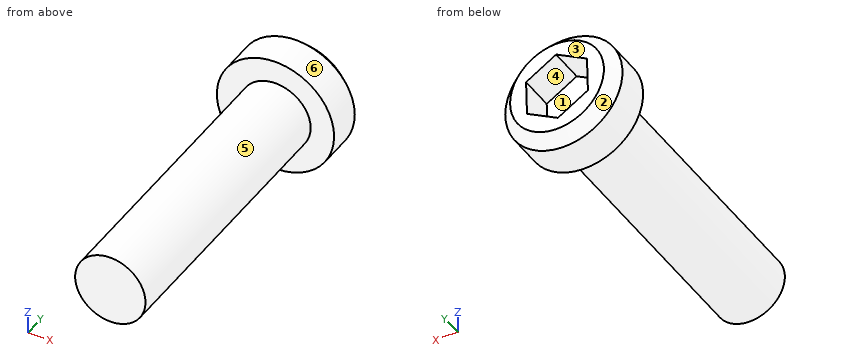
```python
from build123d import *

# Parameters (mm, degrees)
SKETCH1_R           = 1.5
BOSS_EXTRUDE1_DEPTH = 12
SKETCH2_R           = 2.5
BOSS_EXTRUDE2_DEPTH = 2
CHAMFER1_SIZE       = 0.5
CUT_EXTRUDE1_DEPTH  = 1.5


with BuildPart() as part:
    # Sketch1 → Boss-Extrude1 (new body)
    with BuildSketch(Plane(origin=(0, 0, 0), x_dir=(1, 0, 0), z_dir=(0, 1, 0))):
        with Locations((-74.537838868, 155.62707166)):
            Circle(SKETCH1_R)
    extrude(amount=-BOSS_EXTRUDE1_DEPTH)

    # Sketch2 → Boss-Extrude2 (add)
    with BuildSketch(Plane(origin=(0, 0, 0), x_dir=(1, 0, 0), z_dir=(0, 1, 0))):
        with Locations((-74.537838868, 155.62707166)):
            Circle(SKETCH2_R)
    extrude(amount=BOSS_EXTRUDE2_DEPTH)

    # Chamfer1
    chamfer1_edges = [part.edges().sort_by_distance(p)[0] for p in [
        (-77.037838868, 2, -155.62707166),
    ]]
    chamfer(chamfer1_edges, length=CHAMFER1_SIZE)

    # Sketch3 → Cut-Extrude1 (cut)
    with BuildSketch(Plane(origin=(0, 2, 0), x_dir=(1, 0, 0), z_dir=(0, 1, 0))):
        Polygon((-73.219689644, 154.911192742), (-73.258794928, 156.410682915), (-74.576944151, 157.126561832), (-75.855988091, 156.342950577), (-75.816882808, 154.843460404), (-74.498733584, 154.127581487), align=None)
    extrude(amount=-CUT_EXTRUDE1_DEPTH, mode=Mode.SUBTRACT)


solid = part.part
```
CAD build for the part. Positions are in the model's coordinates, mm. Face numbers are marked on the shaded views. A direction names the side the tool comes from. Round coordinates to 2 decimals unless told otherwise and drop trailing zeros. Loops run counter-clockwise (first coordinate to the right, second up) from the corner with the lowest first, then second, coordinate; pieces in that order, holes last. Notation, with made-up numbers: M 25.5,49.25 L 49.5,49.25 A27 cw 49.5,85.25 Z; hole C -5.75,32.5 d1. An arc over 180 degrees is marked long. Use a Markdown table: item, result. Add a question column.
(1) Cut at A-A (y = -8.75). Give the cut face in (x, z), and give its area (3 significant figures).
(2) Flat gauge pins, fed straight in: pin 1 (1.5 mm diameter, centred on x = -75.5, y = -8.5, fed in from -Z); pin 2 (1.5 mm diameter, centred on y = -2, z = -156, fed in from +X); pin 3 (2 mm diameter, centred on x = -73.5, y = -9, fed in from +Z). Where does each tip first touch, or does it go through?
(3) Drill centre lines: line 1 (Y direction, x = -73.9, z = -157.05); line 2 (X direction, y = -6, z = -155.7); line 3 (Y direction, x = -76.65, z = -156.8). Where is each one in solid material? Low to high.
(4) Which spindle directions (+Z, -Z, +X, -X, +Y, -Y) get a long thin tool onto all of the face, cutting with end or side? Do the marked faces 4, 5 and 6. Say none if no direction does.
(5) Pull direction X, two halves, no side cores. Call the marked faces 1, 2 and 3: +X half, -X half, draft (parallel to the pull), parting line (faces both ways), or undercut.
Geometry says:
| question | item | result |
|---|---|---|
| 1 | outline | C -74.54,-155.63 d3 |
| 1 | area | 7.07 mm² |
| 2 | pin 1 | stops at z = -157.11 |
| 2 | pin 2 | stops at x = -73.04 |
| 2 | pin 3 | stops at z = -154.13 |
| 3 | line 1 | y = 0 to 2 |
| 3 | line 2 | x = -76.04 to -73.04 |
| 3 | line 3 | y = 0 to 1.58 |
| 4 | face 4 | +Y |
| 4 | face 5 | -Y |
| 4 | face 6 | +Y, -Y |
| 5 | face 1 | undercut |
| 5 | face 2 | parting line |
| 5 | face 3 | draft |
